from build123d import *

# Parameters (mm, degrees)
BOSS_EXTRUDE1_DEPTH     = 150
SKETCH2_R               = 1.25
CUT_EXTRUDE1_DEPTH      = 10
SKETCH5_R               = 1.25
CUT_EXTRUDE2_DEPTH      = 1
CUT_EXTRUDE2_DEPTH_BACK = 19
SKETCH7_R               = 1.25
CUT_EXTRUDE3_DEPTH      = 2


with BuildPart() as part:
    # Sketch1 → Boss-Extrude1 (new body)
    with BuildSketch(Plane(origin=(0, 0, 0), x_dir=(1, 0, 0), z_dir=(0, 1, 0))):
        Polygon((-7, 4.5), (-7, -2.5), (7, -2.5), (7, 4.5), (9, 4.5), (9, -4.5), (-9, -4.5), (-9, 4.5), align=None)
    extrude(amount=BOSS_EXTRUDE1_DEPTH)

    # Sketch2 → Cut-Extrude1 (cut)
    with BuildSketch(Plane(origin=(0, 0, 2.5), x_dir=(-1, 0, 0), z_dir=(0, 0, -1))):
        with Locations((-2.5, 5)):
            Circle(SKETCH2_R)
        with Locations((2.5, 5)):
            Circle(SKETCH2_R)
        with Locations((2.5, 145)):
            Circle(SKETCH2_R)
        with Locations((-2.5, 145)):
            Circle(SKETCH2_R)
    extrude(amount=-CUT_EXTRUDE1_DEPTH, mode=Mode.SUBTRACT)

    # Sketch5 → Cut-Extrude2 (cut, two sides)
    with BuildSketch(Plane(origin=(9, 0, 0), x_dir=(0, 0, -1), z_dir=(1, 0, 0))) as cut_extrude2_sk:
        with Locations((1, 110.5)):
            Circle(SKETCH5_R)
        with Locations((1, 104.5)):
            Circle(SKETCH5_R)
        with Locations((1, 40.5)):
            Circle(SKETCH5_R)
        with Locations((1, 34.5)):
            Circle(SKETCH5_R)
    extrude(amount=CUT_EXTRUDE2_DEPTH, mode=Mode.SUBTRACT)
    extrude(cut_extrude2_sk.sketch, amount=-CUT_EXTRUDE2_DEPTH_BACK, mode=Mode.SUBTRACT)

    # Sketch7 → Cut-Extrude3 (cut)
    with BuildSketch(Plane.XY.offset(4.5)):
        with Locations((-4, 115)):
            Circle(SKETCH7_R)
        with Locations((4, 115)):
            Circle(SKETCH7_R)
    extrude(amount=-CUT_EXTRUDE3_DEPTH, mode=Mode.SUBTRACT)


solid = part.part
Geometry check sheet. Reference: the model listing, model coordinates, mm. A direction names the side the tool comes from. Give positions to 0.01 mm unless a question says otherwise; leave off trailing zeros. Loops run counter-clockwise (first coordinate to the right, second up) from the corner with the lowest first, then second, coordinate; pieces in that order, holes last. Notation, with made-up numbers: (-32.75, 52.25) -> (-13.75, 52.25) arc R22 ccw to (-13.75, 71.25) -> close; hole circle Ø7 at (65, -9.75). An arc over 180 degrees is marked (long way). Answer in a Markdown table with one row per item. Add a question column.
1) Material ranges on probe 1 along Y at (x, z) = (7.75, -1); probe 2 along X at (y, z) = (145, 3.4); probe 3 along Y at (x, z) = (-2.5, 3), recorded low to high. Write a range as from..to.
2) Gauge pin test, flat ends, axial feed: P1, Ø4, axis at x = 3, y = 94.5, coming from the -Z side; P2, Ø3, axis at y = 104.5, z = -1, coming from the +X side. Record the tip position at first contact, or that the pin passes through.
3) Cross-section at B-B on y = 20. Record the boundary of the cut face in (x, z), and give its area (3 significant figures).
4) Draft check along X on faces 1 (the face through (-4.16, 116.24, 3.51)), 2 (the face through (0, 74, 2.5)), 3 (the face through (-7.99, 111.74, -0.84)), 4 (the face through (-9, 74, 0)). Enter one of: pulls with the +X half, pulls with the -X half, needs draft (parallel to the pull), parting line crosses it, or undercut.
5) Cross-section at A-A on y = 145. Record the boundary of the cut face in (x, z).
6) Set-up check for faces 5 (the face through (-7, 74, -1)), 6 (the face through (3.84, 116.24, 3.51)): record each of +Z, -Z, +X, -X, +Y, -Y from which the full face is reachable in a straight line by a thin tool's end or side.
7) Cross-section at C-C on z = -1. State how many separate pieces and enclosed holes the cut face has, and give its area (3 significant figures).
Outcome:
| question | item | result |
|---|---|---|
| 1 | probe 1 | y = 0..33.25, 35.75..39.25, 41.75..103.25, 105.75..109.25, 111.75..150 |
| 1 | probe 2 | x = -9..-3.75, -1.25..1.25, 3.75..9 |
| 1 | probe 3 | y = 0..3.75, 6.25..143.75, 146.25..150 |
| 2 | P1 | stops at z = 2.5 |
| 2 | P2 | stops at x = 9 |
| 3 | outline | (-9, -4.5) -> (-7, -4.5) -> (-7, 2.5) -> (7, 2.5) -> (7, -4.5) -> (9, -4.5) -> (9, 4.5) -> (-9, 4.5) -> close |
| 3 | area | 64.0 mm^2 |
| 4 | face 1 | undercut |
| 4 | face 2 | undercut |
| 4 | face 3 | needs draft |
| 4 | face 4 | pulls with the -X half |
| 5 | outline | (-9, -4.5) -> (-7, -4.5) -> (-7, 2.5) -> (-3.75, 2.5) -> (-3.75, 4.5) -> (-9, 4.5) -> close; (-1.25, 2.5) -> (1.25, 2.5) -> (1.25, 4.5) -> (-1.25, 4.5) -> close; (3.75, 2.5) -> (7, 2.5) -> (7, -4.5) -> (9, -4.5) -> (9, 4.5) -> (3.75, 4.5) -> close |
| 6 | face 5 | -Z, +Y, -Y |
| 6 | face 6 | +Z, -Z |
| 7 | separate pieces | 10 |
| 7 | enclosed holes | 0 |
| 7 | area | 560 mm^2 |
